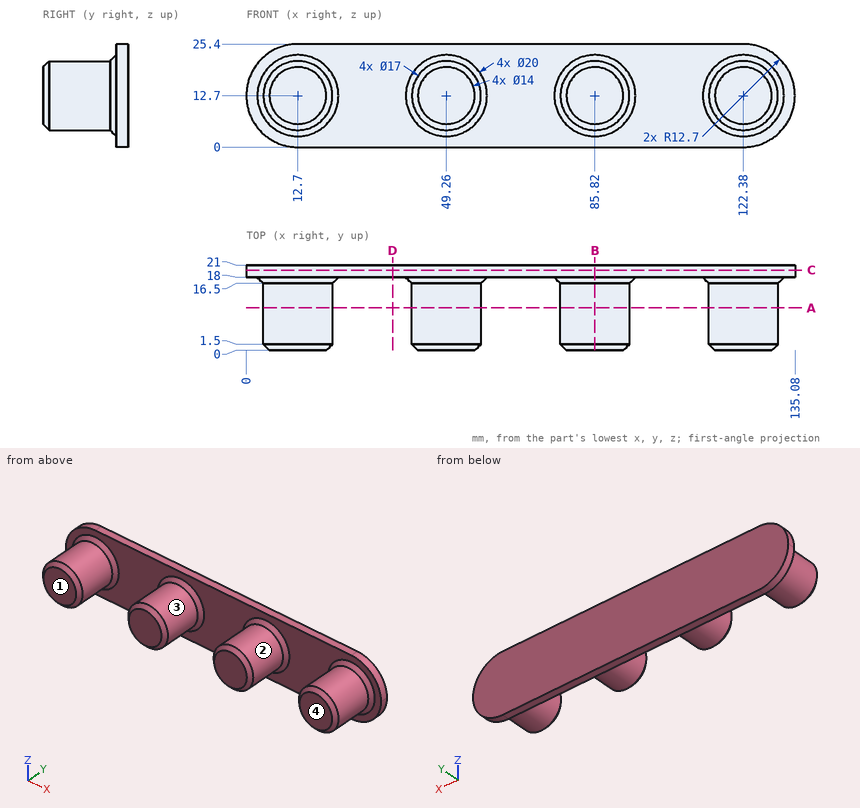
Geometry check sheet. Reference: drawing and pictorial views, mm from the part's lowest x, y, z. A direction names the side the tool comes from. Coordinates: 2 decimals unless noted, no trailing zeros. Loops run counter-clockwise (first coordinate to the right, second up) from the corner with the lowest first, then second, coordinate; pieces in that order, holes last. Notation, with made-up numbers: (86, 2) -> (141, 2) arc R21 cw to (141, 33) -> close; hole circle Ø6 at (-37.75, 53.25). An arc over 180 degrees is marked (long way). Put each result on its own line as item: value.
1) Cross-section at D-D on x = 36. Record the boundary of the cut face in (y, z), plus the area to 3 significant figures.
Result set:
outline: (18, 0) -> (21, 0) -> (21, 25.4) -> (18, 25.4) -> close
area: 76.2 mm^2
2) Tool access check on the marked faces 1 and 2. Record the directions out of +Z, -Z, +X, -X, +Y, -Y that give a thin tool (end or side, any length) a straight path to the whole face; none if there is none.
Result set:
face 1: +Z, -Z, +X, -X, -Y
face 2: -Y
3) Cross-section at A-A on y = 10.5. Record the boundary of the cut face in (x, z), plus the area to 3 significant figures.
Result set:
outline: circle Ø17 at (12.7, 12.7); circle Ø17 at (49.26, 12.7); circle Ø17 at (85.82, 12.7); circle Ø17 at (122.38, 12.7)
area: 908 mm^2
4) Release check for a two-part mould opening along X. For the marked faces 3 and 4 record: released by +X, released by -X, zero draft, split by the parting line, or undercut.
Result set:
face 3: undercut
face 4: zero draft
5) Cross-section at C-C on y = 19.75. Record the boundary of the cut face in (x, z), plus the area to 3 significant figures.
Result set:
outline: (12.7, 0) -> (122.38, 0) arc R12.7 ccw to (122.38, 25.4) -> (12.7, 25.4) arc R12.7 ccw to start
area: 3,290 mm^2
6) Gauge pin test, flat ends, axial feed: pin 1 Ø1 at (x, z) = (68, 21.5) entering from -Y; pin 2 Ø5 at (y, z) = (13, 5.5) entering from +X; pin 3 Ø10 at (x, y) = (76, 12.5) entering from -Z. Record the tip position at first contact, or that the pin passes through.
Result set:
pin 1: stops at y = 18
pin 2: stops at x = 129.46
pin 3: stops at z = 5.7
7) Thickness scan on line 1 (X direction, y = 9, z = 12.25); line 2 (X direction, y = 10, z = 5.5); line 3 (Y direction, x = 96.5, z = 9.5). Record the ranges inside material, lowest first.
Result set:
line 1: x = 4.21 to 21.19, 40.77 to 57.75, 77.33 to 94.31, 113.89 to 130.87
line 2: x = 8.18 to 17.22, 44.74 to 53.78, 81.3 to 90.34, 117.86 to 126.9
line 3: y = 18 to 21
8) Cross-section at B-B on x = 85.82. Record the boundary of the cut face in (y, z).
Result set:
outline: (0, 5.7) -> (1.5, 4.2) -> (16.5, 4.2) -> (18, 2.7) -> (18, 0) -> (21, 0) -> (21, 25.4) -> (18, 25.4) -> (18, 22.7) -> (16.5, 21.2) -> (1.5, 21.2) -> (0, 19.7) -> close
